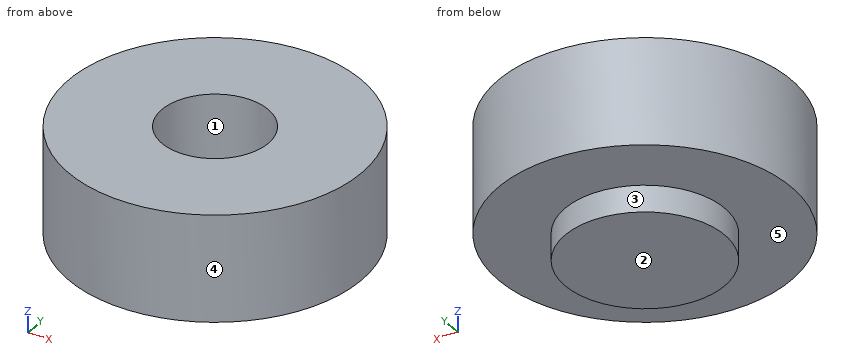
```python
from build123d import *

# Parameters (mm, degrees)
F0_R     = 2.75
F1_DEPTH = 8
F2_R     = 2.75
F2_R_2   = 1.5
F3_DEPTH = 6
F4_R     = 1
F5_DEPTH = 2
F6_R     = 1.5
F7_DEPTH = 5.5


with BuildPart() as f1:
    # F0 (on Top) → F1 (new body)
    with BuildSketch(Plane.XY):
        Circle(F0_R)
    extrude(amount=F1_DEPTH)

    # F2 (on face) → F3 (cut)
    with BuildSketch(Plane(origin=(0, 0, 0), x_dir=(1, 0, 0), z_dir=(0, 0, -1))):
        Circle(F2_R)
        Circle(F2_R_2, mode=Mode.SUBTRACT)
    extrude(amount=-F3_DEPTH, mode=Mode.SUBTRACT)

    # F4 (on face) → F5 (cut)
    with BuildSketch(Plane.XY.offset(8)):
        Circle(F4_R)
    extrude(amount=-F5_DEPTH, mode=Mode.SUBTRACT)

    # F6 (on face) → F7 (cut)
    with BuildSketch(Plane(origin=(0, 0, 0), x_dir=(1, 0, 0), z_dir=(0, 0, -1))):
        Circle(F6_R)
    extrude(amount=-F7_DEPTH, mode=Mode.SUBTRACT)


solid = f1.part
```
Can you work these out from the model? Positions are in its coordinate system, mm. Face numbers are marked on the shaded views. A direction names the side the tool comes from. Coordinates: 2 decimals unless noted, no trailing zeros. Order: outer loops, then holes, each group sorted by start corner. A loop starts at its lowest first (then second) coordinate and runs counter-clockwise, first axis right, second up. Notation, with made-up numbers: (-9, -1.5) -> (44, -1.5) arc R16 ccw to (44, 21.5) -> close; hole circle Ø3 at (-22.75, -27). An arc over 180 degrees is marked (long way). Write each question's results on one line, items separated by ' | '.
Item 1: If I drill on line 1 along Y through (x, z) = (0, 6.7); line 2 along Z through (x, y) = (0, 2.05); line 3 along X through (y, z) = (0.1, 7.5), over which ranges is the centre line in solid material (lowest first)?
Results are:
line 1: -2.75 to -1, 1 to 2.75 | line 2: 6 to 8 | line 3: -2.75 to -0.99, 0.99 to 2.75
Item 2: I want a section at C-C, the plane z = 7.55. Write out the boundary of the cut face in (x, y).
Results are:
outline: circle Ø5.5 at (0, 0); hole circle Ø2 at (0, 0)
Item 3: Which directions (+Z, -Z, +X, -X, +Y, -Y) give clear straight access to the entire face, cutting with the end or side of a thin tool? Please do the marked faces 4 and 5.
Results are:
face 4: +Z, -Z | face 5: -Z
Item 4: I want a section at D-D, the plane y = -1.15. Write out the boundary of the cut face in (x, z).
Results are:
outline: (-2.5, 6) -> (-0.96, 6) -> (-0.96, 5.5) -> (0.96, 5.5) -> (0.96, 6) -> (2.5, 6) -> (2.5, 8) -> (-2.5, 8) -> close
Item 5: If we mould it in two halves opening along X, with no side actions, what happens to the marked faces 1, 2 and 3? For each: +X half, -X half, draft (parallel to the pull), parting line (faces both ways), or undercut.
Results are:
face 1: undercut | face 2: draft | face 3: parting line
Item 6: I'm going to push flat-ended pins straight in: pin 1 Ø1.6 at (x, y) = (0, 0) entering from +Z; pin 2 Ø1.5 at (y, z) = (-1.5, 7.5) entering from +X; pin 3 Ø1.5 at (x, z) = (-2, 6.5) entering from -Y. Where does each tip first touch, or does it pass through?
Results are:
pin 1: z = 6 | pin 2: x = 2.65 | pin 3: y = -2.45
Item 7: I want a section at A-A, the plane y = 0. Write out the boundary of the cut face in (x, z), then the cut area to 3 significant figures.
Results are:
outline: (-2.75, 6) -> (-1.5, 6) -> (-1.5, 5.5) -> (1.5, 5.5) -> (1.5, 6) -> (2.75, 6) -> (2.75, 8) -> (1, 8) -> (1, 6) -> (-1, 6) -> (-1, 8) -> (-2.75, 8) -> close | area: 8.50 mm²
